from build123d import *

# Parameters (mm, degrees)
F0_W     = 106.934
F0_H     = 31.75
F0_W_2   = 100.584
F0_H_2   = 25.4
F1_DEPTH = 13.97
F2_DEPTH = 3.175
F3_W     = 106.934
F3_H     = 31.75
F3_W_2   = 103.759
F3_H_2   = 28.575
F4_DEPTH = 6.35
F5_R     = 2.54


with BuildPart() as f1:
    # F0 (on Top) → F1 (new body)
    with BuildSketch(Plane.XY):
        with Locations((50.292, 12.7)):
            Rectangle(F0_W, F0_H)
        with Locations((50.292, 12.7)):
            Rectangle(F0_W_2, F0_H_2, mode=Mode.SUBTRACT)
    extrude(amount=F1_DEPTH)

    # F0 (on Top) → F2 (join)
    with BuildSketch(Plane.XY):
        with Locations((50.292, 12.7)):
            Rectangle(F0_W_2, F0_H_2)
    extrude(amount=F2_DEPTH)

    # F3 (on face) → F4 (cut)
    with BuildSketch(Plane.XY.offset(13.97)):
        with Locations((50.292, 12.7)):
            Rectangle(F3_W, F3_H)
        with Locations((50.292, 12.7)):
            Rectangle(F3_W_2, F3_H_2, mode=Mode.SUBTRACT)
    extrude(amount=-F4_DEPTH, mode=Mode.SUBTRACT)

    # F5
    f5_edges = [f1.edges().sort_by_distance(p)[0] for p in [
        (-1.5875, -1.5875, 10.795),
        (-3.175, -3.175, 3.81),
        (-1.5875, 26.9875, 10.795),
        (-3.175, 28.575, 3.81),
        (102.1715, -1.5875, 10.795),
        (103.759, -3.175, 3.81),
        (103.759, 28.575, 3.81),
        (102.1715, 26.9875, 10.795),
    ]]
    fillet(f5_edges, radius=F5_R)


solid = f1.part
Work out the finished part from the listing and answer in its coordinate system (mm). A direction names the side the tool comes from. Round coordinates to 2 decimals unless told otherwise and drop trailing zeros. Loops run counter-clockwise (first coordinate to the right, second up) from the corner with the lowest first, then second, coordinate; pieces in that order, holes last. Notation, with made-up numbers: (66, -12) - (113, -12) arc R29 cw to (113, 13) - close; hole circle Ø6 at (-33, 17). An arc over 180 degrees is marked (long way). Use one line per item in the form item = value. Start each with the question number.
(1) Find section A-A on z = 4.25. Determine the outline of the cut face in (x, y) (3 decimals).
(2) Consider line 1 (Y direction, x = 16.5, z = 12.75); line 2 (X direction, y = 12.5, z = 4.5) (3 decimals); line 3 (Y direction, x = 46, z = 5.5) (3 decimals). Determine where each line is inside the solid, lowest interval first.
(3) Find section C-C on x = 25. Determine the outline of the cut face in (y, z) (1 decimal), and give its area (3 significant figures).
(4) Find section B-B on y = 17. Determine the outline of the cut face in (x, z) (1 decimal), and give its area (3 significant figures).
(5) Find section D-D on z = 11.25. Determine the outline of the cut face in (x, y).
(6) Flat-ended cylindrical pins translate along their axes: P1, Ø1, axis at x = 80.5, z = 10.5, coming from the -Y side; P2, Ø1, axis at y = 11.5, z = 10, coming from the -X side; P3, Ø3, axis at x = 38, z = 12.5, coming from the +Y side. Find the tip coordinate at first contact, or state that the pin passes through.
(7) Determine the mould class of faces 6 (the face through (0, 13, 8)), 7 (the face through (-3.175, 13, 4)), 8 (the face through (50, 13, 0)), 9 (the face through (100.584, 13, 8)) for opening direction X: +X half, -X half, draft (parallel to the pull), parting line (faces both ways), or undercut.
(8) Which of the six approach directions +Z, -Z, +X, -X, +Y, -Y give full straight-line access (tool end or side, diameter ignored) to faces 1 (the face through (101.45, 26.22, 10.75)), 2 (the face through (50, -1.588, 11)), 3 (the face through (50, 26.987, 11)), 4 (the face through (-1.587, 13, 11)), 5 (the face through (50, 0, 8))?
Answer list:
q1.outline = (-3.175, -0.635) arc R2.54 ccw to (-0.635, -3.175) - (101.219, -3.175) arc R2.54 ccw to (103.759, -0.635) - (103.759, 26.035) arc R2.54 ccw to (101.219, 28.575) - (-0.635, 28.575) arc R2.54 ccw to (-3.175, 26.035) - close; hole (0, 0) - (100.584, 0) - (100.584, 25.4) - (0, 25.4) - close
q2.line_1 = -1.59 to 0, 25.4 to 26.99
q2.line_2 = -3.175 to 0, 100.584 to 103.759
q2.line_3 = -3.175 to 0, 25.4 to 28.575
q3.outline = (-3.2, 0) - (28.6, 0) - (28.6, 7.6) - (27, 7.6) - (27, 14) - (25.4, 14) - (25.4, 3.2) - (0, 3.2) - (0, 14) - (-1.6, 14) - (-1.6, 7.6) - (-3.2, 7.6) - close
q3.area = 149 mm^2
q4.outline = (-3.2, 0) - (103.8, 0) - (103.8, 7.6) - (102.2, 7.6) - (102.2, 14) - (100.6, 14) - (100.6, 3.2) - (0, 3.2) - (0, 14) - (-1.6, 14) - (-1.6, 7.6) - (-3.2, 7.6) - close
q4.area = 388 mm^2
q5.outline = (-1.59, 0.95) arc R2.54 ccw to (0.95, -1.59) - (99.63, -1.59) arc R2.54 ccw to (102.17, 0.95) - (102.17, 24.45) arc R2.54 ccw to (99.63, 26.99) - (0.95, 26.99) arc R2.54 ccw to (-1.59, 24.45) - close; hole (0, 0) - (100.58, 0) - (100.58, 25.4) - (0, 25.4) - close
q6.P1 = -1.59
q6.P2 = -1.59
q6.P3 = 26.99
q7.face_6 = undercut
q7.face_7 = -X half
q7.face_8 = draft
q7.face_9 = undercut
q8.face_1 = +Z, +X, +Y
q8.face_2 = +Z, +X, -X, -Y
q8.face_3 = +Z, +X, -X, +Y
q8.face_4 = +Z, -X, +Y, -Y
q8.face_5 = +Z
